Autodesk Inventor part; units mm, degrees
ref_plane "YZ Plane" through (0, 0, 0) normal (1, 0, 0) x (0, 1, 0)
ref_plane "XZ Plane" through (0, 0, 0) normal (0, 1, 0) x (-1, 0, 0)
ref_plane "XY Plane" through (0, 0, 0) normal (0, 0, 1) x (1, 0, 0)
sketch "Sketch1" plane through (0, 0, 0) normal (0, 1, 0) x (-1, 0, 0)
  line L0 (19.05, 22.8956) -> (38.1, 22.8956)
  line L1 (38.1, 22.8956) -> (19.05, 22.8956)
  line L2 (19.05, -22.8956) -> (38.1, -22.8956)
  line L3 (38.1, -22.8956) -> (38.1, 22.8956)
  line L4 (38.1, 22.8956) -> (19.05, 22.8956)
  line L5 (19.05, 22.8956) -> (19.05, -22.8956)
  line L6 (38.1, 22.8956) -> (28.575, 22.8956)
  circle A0 centre (28.575, 11.4465) radius 4.445
  circle A1 centre (28.575, -11.4516) radius 4.445
  dimension "d6" = 45.7911
  dimension "d7" = 19.05
  dimension "d8" = 19.05
  dimension "d9" = 9.525
  dimension "d13" = 8.89
extrude "Extrusion1" add sketch "Sketch1" along normal blind 7.112
properties part number "BracketOfTheBracket"
Geometry: final body of the model. Coordinates: model frame, mm. Coordinates: 2 decimals unless noted, no trailing zeros. Order: outer loops, then holes, each group sorted by start corner. A loop starts at its lowest first (then second) coordinate and runs counter-clockwise, first axis right, second up.
1) Section C-C (y = 2.5). Give the number of separate pieces and of enclosed holes in the cut face, then the cut area to 3 significant figures.
Result sheet:
separate pieces: 1
enclosed holes: 2
area: 748 mm2
2) Ray query, probe 1 along Z at (x, y) = (-28.75, 3.75); probe 2 along Z at (x, y) = (-31.75, 4.75); probe 3 along X at (y, z) = (6.5, -8). Return the intervals inside material, ascending.
Result sheet:
probe 1: z = -22.9 to -15.89, -7.01 to 7, 15.89 to 22.9
probe 2: z = -22.9 to -14.56, -8.34 to 8.34, 14.56 to 22.9
probe 3: x = -38.1 to -31.38, -25.77 to -19.05
3) Section A-A (z = -14). Return loops of the section in (x, y).
Result sheet:
outline: (-38.1, 0) - (-32.22, 0) - (-32.22, 7.11) - (-38.1, 7.11) - close; (-24.93, 0) - (-19.05, 0) - (-19.05, 7.11) - (-24.93, 7.11) - close
4) Section D-D (x = -26.5). Return loops of the section in (y, z), then the cut area to 3 significant figures.
Result sheet:
outline: (0, -22.9) - (7.11, -22.9) - (7.11, -15.38) - (0, -15.38) - close; (0, -7.52) - (7.11, -7.52) - (7.11, 7.52) - (0, 7.52) - close; (0, 15.38) - (7.11, 15.38) - (7.11, 22.9) - (0, 22.9) - close
area: 214 mm2
5) Section B-B (x = -29.75). Return loops of the section in (y, z), then the cut area to 3 significant figures.
Result sheet:
outline: (0, -22.9) - (7.11, -22.9) - (7.11, -15.74) - (0, -15.74) - close; (0, -7.16) - (7.11, -7.16) - (7.11, 7.16) - (0, 7.16) - close; (0, 15.73) - (7.11, 15.73) - (7.11, 22.9) - (0, 22.9) - close
area: 204 mm2
6) Draft query along Z for faces 1 (the cylindrical face through (-24.134, 3.506, -11.647)), 2 (the flat face through (-28, 4, 22.896)), 3 (the flat face through (-28, 0, 0)). Return one class per face: released by +Z, released by -Z, zero draft, split by the parting line, or undercut.
Result sheet:
face 1: undercut
face 2: released by +Z
face 3: zero draft
